```python
from build123d import *

# Parameters (mm, degrees)
SKETCH_4_R          = 1.75
CUT_EXTRUDE_1_DEPTH = 10
CUT_EXTRUDE_2_DEPTH = 1
CHAMFER_1_SIZE      = 0.5


with BuildPart() as part:
    # 草图3 → 旋转1 (revolve)
    with BuildSketch(Plane(origin=(0, 0, 0), x_dir=(0, 0, -1), z_dir=(1, 0, 0)), mode=Mode.PRIVATE) as revolve_1_sk:
        Polygon((-7.5, 0), (0, 0), (0, -4), (-4.5, -4), (-16, -50), (-20, -50), align=None)
    revolve(revolve_1_sk.sketch.rotate(Axis((0, 28.450677981, 0), (0, 1, 0)), 180), axis=Axis((0, 28.450677981, 0), (0, 1, 0)))

    # 草图4 → 切除-拉伸1 (cut)
    with BuildSketch(Plane(origin=(0, 0, 0), x_dir=(1, 0, 0), z_dir=(0, 1, 0))):
        with Locations(Location((0, 0, 0), (0, 0, 270))):
            Circle(SKETCH_4_R)
    extrude(amount=-CUT_EXTRUDE_1_DEPTH, mode=Mode.SUBTRACT)

    # 草图5 → 切除-拉伸2 (cut)
    with BuildSketch(Plane(origin=(0, 0, 0), x_dir=(1, 0, 0), z_dir=(0, 1, 0))):
        Polygon((3.5, 0), (1.75, 3.031088913), (-1.75, 3.031088913), (-3.5, 0), (-1.75, -3.031088913), (1.75, -3.031088913), align=None)
    extrude(amount=-CUT_EXTRUDE_2_DEPTH, mode=Mode.SUBTRACT)

    # 倒角1
    chamfer_1_edges = [part.edges().sort_by_distance(p)[0] for p in [
        (0, -4, -1.75),
    ]]
    chamfer(chamfer_1_edges, length=CHAMFER_1_SIZE)


solid = part.part
```
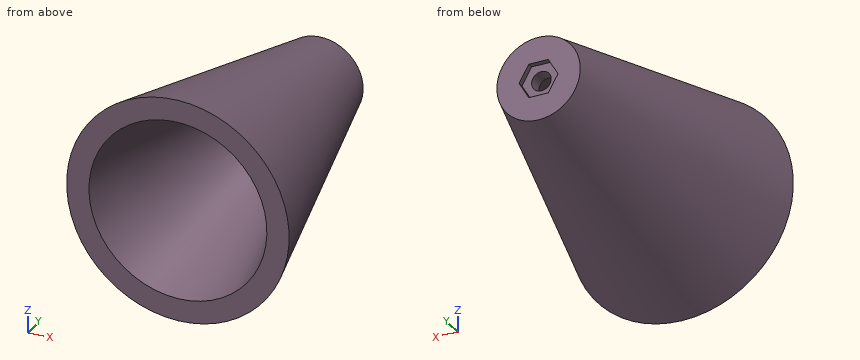
The listing builds one solid part. Answer for the finished solid, in the listing's coordinates (mm). Coordinates: 2 decimals unless noted, no trailing zeros. Loops run counter-clockwise (first coordinate to the right, second up) from the corner with the lowest first, then second, coordinate; pieces in that order, holes last. Notation, with made-up numbers: (-25.75, -32.75) -> (3.25, -32.75) arc R14 ccw to (3.25, -5.75) -> close; hole circle Ø11 at (51, -12). An arc over 180 degrees is marked (long way). Return JSON: item names as keys, results as strings. Group by question number.
(1) A cutting plane is placed at A-A on x = 0. Write down the section's boundary in (y, z).
(2) Find the intervals of material crossed by probe 1 along X at (y, z) = (-2, 0); probe 2 along Z at (x, y) = (9, -28.5); probe 3 along X at (y, z) = (-23.5, -8), in increasing order. Write a range as from..to.
(3) A cutting plane is placed at C-C on y = -13.5. Write down the section's boundary in (x, z) (3 decimals), and give its area (3 significant figures).
(4) A cutting plane is placed at B-B on y = -40. Write down the section's boundary in (x, z), and give its area (3 significant figures).
(5) Given pin 1 Ø0.5 at (x, y) = (0, -0.5) entering from +Z; pin 2 Ø5.5 at (x, z) = (0, 0) entering from +Y; pin 3 Ø0.8 at (x, y) = (-1, -0.5) entering from -Z, each flat-ended and moving along its own axis, determine where each tip first touches the part or whether it passes through.
The answers:
{
 "1": {"outline": "(-50, -20) -> (0, -7.5) -> (0, -3.03) -> (-1, -3.03) -> (-1, -1.75) -> (-3.5, -1.75) -> (-4, -2.25) -> (-4, -4.5) -> (-50, -16) -> close; (-50, 16) -> (-4, 4.5) -> (-4, 2.25) -> (-3.5, 1.75) -> (-1, 1.75) -> (-1, 3.03) -> (0, 3.03) -> (0, 7.5) -> (-50, 20) -> close"},
 "2": {"probe 1": "x = -8..-1.75, 1.75..8", "probe 2": "z = -11.53..-5.65, 5.65..11.53", "probe 3": "x = -10.72..-4.89, 4.89..10.72"},
 "3": {"outline": "circle Ø21.75 at (0, 0); hole circle Ø13.75 at (0, 0)", "area": "223 mm^2"},
 "4": {"outline": "circle Ø35 at (0, 0); hole circle Ø27 at (0, 0)", "area": "390 mm^2"},
 "5": {"pin 1": "stops at z = 7.69", "pin 2": "stops at y = -1", "pin 3": "stops at z = -7.67"}
}
